Check sheet for the modelled part. Datum: model origin and axes. Units: mm. Coordinates: 2 decimals unless noted, no trailing zeros. Order: outer loops, then holes, each group sorted by start corner. A loop starts at its lowest first (then second) coordinate and runs counter-clockwise, first axis right, second up.
from build123d import *

# Parameters (mm, degrees)
SKETCH1_W           = 91.267371632
SKETCH1_H           = 49.068479372
BOSS_EXTRUDE1_DEPTH = 10
SKETCH2_R           = 6.742418782
CUT_EXTRUDE2_DEPTH  = 10


with BuildPart() as part:
    # Sketch1 → Boss-Extrude1 (new body)
    with BuildSketch(Plane(origin=(0, 0, 0), x_dir=(1, 0, 0), z_dir=(0, 1, 0))):
        with Locations((-64.279707977, 31.526497996)):
            Rectangle(SKETCH1_W, SKETCH1_H)
    extrude(amount=BOSS_EXTRUDE1_DEPTH)

    # Sketch2 → Cut-Extrude2 (cut)
    with BuildSketch(Plane(origin=(0, 10, 0), x_dir=(1, 0, 0), z_dir=(0, 1, 0))):
        with Locations((-95.875303576, 30.408499998)):
            Circle(SKETCH2_R)
    cut_extrude2 = extrude(amount=-CUT_EXTRUDE2_DEPTH, mode=Mode.SUBTRACT)

    # Mirror1: Cut-Extrude2 across plane
    add(cut_extrude2.mirror(Plane.ZY.offset(64.279707977)), mode=Mode.SUBTRACT)


solid = part.part
(1) Thickness scan on probe 1 along Z at (x, y) = (-33, 4.5); probe 2 along X at (y, z) = (1.75, -35); probe 3 along X at (y, z) = (3.75, -36.5) (3 decimals). Record the ranges inside material, lowest first.
Filled in:
probe 1: z = -56.06 to -37.14, -23.67 to -6.99
probe 2: x = -109.91 to -100.81, -90.94 to -37.62, -27.75 to -18.65
probe 3: x = -109.913 to -98.766, -92.985 to -35.574, -29.794 to -18.646
(2) Go/stop test with a flat-tipped pin: P1, Ø8, axis at x = -95.88, z = -30.41, coming from the +Y side. Record where the tip stops, or that it passes through.
Filled in:
P1: passes through
(3) Cross-section at C-C (y = 3). Enter the section's corners in (x, z), and give its area (3 significant figures).
Filled in:
outline: (-109.91, -56.06) - (-18.65, -56.06) - (-18.65, -6.99) - (-109.91, -6.99) - close; hole circle Ø13.48 at (-95.88, -30.41); hole circle Ø13.48 at (-32.68, -30.41)
area: 4,190 mm2
(4) Cross-section at D-D (x = -92). Enter the section's corners in (y, z).
Filled in:
outline: (0, -56.06) - (10, -56.06) - (10, -35.93) - (0, -35.93) - close; (0, -24.89) - (10, -24.89) - (10, -6.99) - (0, -6.99) - close
(5) Cross-section at A-A (z = -31.5). Enter the section's corners in (x, y).
Filled in:
outline: (-109.91, 0) - (-102.53, 0) - (-102.53, 10) - (-109.91, 10) - close; (-89.22, 0) - (-39.34, 0) - (-39.34, 10) - (-89.22, 10) - close; (-26.03, 0) - (-18.65, 0) - (-18.65, 10) - (-26.03, 10) - close
(6) Cross-section at B-B (x = -28.5). Enter the section's corners in (y, z), and give its area (3 significant figures).
Filled in:
outline: (0, -56.06) - (10, -56.06) - (10, -35.7) - (0, -35.7) - close; (0, -25.12) - (10, -25.12) - (10, -6.99) - (0, -6.99) - close
area: 385 mm2
